Could you check a few things on this model? Use its own coordinates, in mm. A direction names the side the tool comes from. Give positions to 0.01 mm unless a question says otherwise; leave off trailing zeros. Order: outer loops, then holes, each group sorted by start corner. A loop starts at its lowest first (then second) coordinate and runs counter-clockwise, first axis right, second up. Notation, with made-up numbers: M 69.5,52 L 88.5,52 A12 cw 88.5,59 Z; hole C -33.75,40 d4. An arc over 180 degrees is marked long. Use a Markdown table: item, result. Add a question column.
Item 1: For faces 4 (the face through (35.821, 4.493, -11.113)), 5 (the face through (43.361, 2, -2)), 6 (the face through (33, 2, -12)), which set-ups out of +Z, -Z, +X, -X, +Y, -Y let a thin tool reach every point of the face, with its end or its side?
Item 2: If I drill on L1, parallel to Z at x = -24.5, y = 2.8; L2, parallel to Z at x = 34, y = 3; L3, parallel to X at y = 0.85, z = 5.5, over which ranges is the centre line in solid material (lowest first)? Write a range as from..to.
Item 3: Suppose I cut it at C-C on y = 1.15. Count the separate pieces of the cut face and the enclosed holes in it, plus the area to 3 significant figures.
Item 4: If we mould it in two halves opening along Z, with no side actions, what happens to faces 1 (the face through (34, 2, 7)), 2 (the face through (42, 2.5, 15)), 3 (the face through (-21.549, 3.455, -13.824))? For each: released by +Z, released by -Z, zero draft, split by the parting line, or undercut.
Item 5: Suppose I cut it at A-A on x = 15.5. Write out the boundary of the cut face in (y, z), plus the area to 3 significant figures.
Item 6: I'm going to push flat-ended pins straight in: pin 1 Ø1 at (x, y) = (34, 3.5) entering from +Z; pin 2 Ø0.8 at (y, z) = (1.5, -14) entering from +X; pin 3 Ø1 at (x, y) = (0.5, 4) entering from -Z. Where does each tip first touch, or does it pass through?
Item 7: Suppose I cut it at B-B on z = -0.5. Write out the boundary of the cut face in (x, y).
from build123d import *

# Parameters (mm, degrees)
SKETCH1_W                = 84.6
SKETCH1_H                = 27
BOSS_EXTRUDE1_DEPTH      = 5
CUT_EXTRUDE1_REACH       = 50.274
BOSS_EXTRUDE3_START      = 2
BOSS_EXTRUDE3_DEPTH      = 2
CUT_EXTRUDE3_START       = -2.5
CUT_EXTRUDE3_DEPTH       = 2.5
CUT_EXTRUDE5_START       = -2.5
CUT_EXTRUDE5_DEPTH       = 46.773999335
BOSS_EXTRUDE4_DEPTH      = 2.5
BOSS_EXTRUDE5_START      = -2.5
BOSS_EXTRUDE5_DEPTH      = 2.5
CUT_EXTRUDE2_OUTLINE_R   = 0.5
CUT_EXTRUDE2_OUTLINE_R_2 = 0.499999992
CUT_EXTRUDE2_DEPTH       = 5
SKETCH15_R               = 0.5
CUT_EXTRUDE6_DEPTH       = 50.255349811
SKETCH16_R               = 0.45
BOSS_EXTRUDE6_DEPTH      = 1


# Read off the part's stored shape, not the designer's step: Cut-Extrude2
with BuildPart() as part:
    # Sketch1 → Boss-Extrude1 (new body)
    with BuildSketch(Plane(origin=(0, 0, 0), x_dir=(1, 0, 0), z_dir=(0, 1, 0))):
        with Locations((3.06331835, 2.23366963)):
            Rectangle(SKETCH1_W, SKETCH1_H)
    extrude(amount=BOSS_EXTRUDE1_DEPTH)

    # Sketch3 → Cut-Extrude1 (cut, up to next)
    with BuildSketch(Plane(origin=(0, 0, 0), x_dir=(1, 0, 0), z_dir=(0, 1, 0)), mode=Mode.PRIVATE) as cut_extrude1_sk1:
        with BuildLine():
            Line((32.919678843, -9.163538235), (-27.280321157, -9.163538235))
            Line((-27.280321157, -9.163538235), (-27.280321157, -7.45100236))
            ThreePointArc((-27.280321157, -7.45100236), (-27.780321157, -6.95100236), (-28.280321157, -7.45100236))
            Line((-28.280321157, -7.45100236), (-28.280321157, -9.262483826))
            Line((-28.280321157, -9.262483826), (-34.233122665, -9.262483826))
            Line((-34.233122665, -9.262483826), (-34.233122665, -4.266133774))
            ThreePointArc((-34.233122665, -4.266133774), (-34.380628165, -3.910023997), (-34.736737941, -3.762518498))
            Line((-34.736737941, -3.762518498), (-37.233015401, -3.762518498))
            Line((-37.233015401, -3.762518498), (-37.233015401, 8.229171698))
            Line((-37.233015401, 8.229171698), (-34.736926038, 8.23003019))
            ThreePointArc((-34.736926038, 8.23003019), (-34.380928238, 8.377596904), (-34.233483972, 8.733645436))
            Line((-34.233483972, 8.733645436), (-34.233483972, 13.729919004))
            Line((-34.233483972, 13.729919004), (-31.31194803, 13.729919004))
            Line((-31.31194803, 13.729919004), (-31.31194803, 12.633776758))
            ThreePointArc((-31.31194803, 12.633776758), (-29.91194803, 11.233776758), (-28.51194803, 12.633776758))
            Line((-28.51194803, 12.633776758), (-28.51194803, 13.730371923))
            Line((-28.51194803, 13.730371923), (-21.508882253, 13.730371923))
            Line((-21.508882253, 13.730371923), (-20.139800412, 10.535595096))
            ThreePointArc((-20.139800412, 10.535595096), (-19.954180397, 10.31357804), (-19.676997597, 10.230415195))
            Line((-19.676997597, 10.230415195), (25.793967371, 10.230415195))
            ThreePointArc((25.793967371, 10.230415195), (26.055680662, 10.259428791), (26.266864173, 10.416709306))
            Line((26.266864173, 10.416709306), (27.639394616, 13.61080525))
            Line((27.639394616, 13.61080525), (34.4513038, 13.61080525))
            Line((34.4513038, 13.61080525), (34.4513038, 12.512891353))
            ThreePointArc((34.4513038, 12.512891353), (35.8513038, 11.112891353), (37.2513038, 12.512891353))
            Line((37.2513038, 12.512891353), (37.2513038, 13.612023992))
            Line((37.2513038, 13.612023992), (40.361611802, 13.612023992))
            Line((40.361611802, 13.612023992), (40.361611802, 8.61576965))
            ThreePointArc((40.361611802, 8.61576965), (40.509053891, 8.259723294), (40.865047712, 8.112154406))
            Line((40.865047712, 8.112154406), (43.361137065, 8.111265408))
            Line((43.361137065, 8.111265408), (43.361137065, -3.763055079))
            Line((43.361137065, -3.763055079), (40.86393165, -3.763055079))
            ThreePointArc((40.86393165, -3.763055079), (40.507821873, -3.910560578), (40.360316374, -4.266670355))
            Line((40.360316374, -4.266670355), (40.360316374, -9.163538235))
            Line((40.360316374, -9.163538235), (34.019678843, -9.163538235))
            Line((34.019678843, -9.163538235), (34.019678843, -7.715606668))
            ThreePointArc((34.019678843, -7.715606668), (33.469678843, -7.165606668), (32.919678843, -7.715606668))
            Line((32.919678843, -7.715606668), (32.919678843, -9.163538235))
        make_face()
    cut_extrude1_tool1 = extrude(cut_extrude1_sk1.sketch, amount=CUT_EXTRUDE1_REACH, mode=Mode.PRIVATE) & part.part
    add(cut_extrude1_tool1.solids().sort_by_distance((3.012517, 0, -1.196465))[0], mode=Mode.SUBTRACT)

    # Sketch3<5> → Boss-Extrude3 (add)
    with BuildSketch(Plane(origin=(0, 0, 0), x_dir=(1, 0, 0), z_dir=(0, 1, 0)).offset(BOSS_EXTRUDE3_START)):
        with BuildLine():
            Line((26.852330657, -9.163538235), (32.919678843, -9.163538235))
            Line((32.919678843, -9.163538235), (32.919678843, -7.715606668))
            ThreePointArc((32.919678843, -7.715606668), (33.469678843, -7.165606668), (34.019678843, -7.715606668))
            Line((34.019678843, -7.715606668), (34.019678843, -9.163538235))
            Line((34.019678843, -9.163538235), (40.360316374, -9.163538235))
            Line((40.360316374, -9.163538235), (40.360316374, -4.950942773))
            Line((40.360316374, -4.950942773), (27.852330657, -4.950942773))
            ThreePointArc((27.852330657, -4.950942773), (27.145223876, -5.243835992), (26.852330657, -5.950942773))
            Line((26.852330657, -5.950942773), (26.852330657, -9.163538235))
        make_face()
        with BuildLine():
            Line((-27.280321157, -9.163538235), (-22.401406955, -9.163538235))
            Line((-22.401406955, -9.163538235), (-22.401406955, -5.777559213))
            ThreePointArc((-22.401406955, -5.777559213), (-22.692236098, -5.07252255), (-23.395560348, -4.777576304))
            Line((-23.395560348, -4.777576304), (-34.233122665, -4.777576304))
            Line((-34.233122665, -4.777576304), (-34.233122665, -9.262483826))
            Line((-34.233122665, -9.262483826), (-28.280321157, -9.262483826))
            Line((-28.280321157, -9.262483826), (-28.280321157, -7.45100236))
            ThreePointArc((-28.280321157, -7.45100236), (-27.780321157, -6.95100236), (-27.280321157, -7.45100236))
            Line((-27.280321157, -7.45100236), (-27.280321157, -9.163538235))
        make_face()
        with BuildLine():
            Line((26.400356299, 10.727366647), (40.361611802, 10.727366647))
            Line((40.361611802, 10.727366647), (40.361611802, 13.612023992))
            Line((40.361611802, 13.612023992), (37.2513038, 13.612023992))
            Line((37.2513038, 13.612023992), (37.2513038, 12.512891353))
            ThreePointArc((37.2513038, 12.512891353), (35.8513038, 11.112891353), (34.4513038, 12.512891353))
            Line((34.4513038, 12.512891353), (34.4513038, 13.61080525))
            Line((34.4513038, 13.61080525), (27.639394616, 13.61080525))
            Line((27.639394616, 13.61080525), (26.400356299, 10.727366647))
        make_face()
        with BuildLine():
            Line((-34.233483972, 13.729919004), (-34.233483972, 10.733923481))
            Line((-34.233483972, 10.733923481), (-20.224791573, 10.733923481))
            Line((-20.224791573, 10.733923481), (-21.508882253, 13.730371923))
            Line((-21.508882253, 13.730371923), (-28.51194803, 13.730371923))
            Line((-28.51194803, 13.730371923), (-28.51194803, 12.633776758))
            ThreePointArc((-28.51194803, 12.633776758), (-29.91194803, 11.233776758), (-31.31194803, 12.633776758))
            Line((-31.31194803, 12.633776758), (-31.31194803, 13.729919004))
            Line((-31.31194803, 13.729919004), (-34.233483972, 13.729919004))
        make_face()
    extrude(amount=BOSS_EXTRUDE3_DEPTH)

    # Sketch13 → Cut-Extrude3 (cut)
    with BuildSketch(Plane(origin=(0, 5, 0), x_dir=(1, 0, 0), z_dir=(0, 1, 0)).offset(CUT_EXTRUDE3_START)):
        with BuildLine():
            Line((-22.367370549, 15.73366963), (-20.139800412, 10.535595096))
            ThreePointArc((-20.139800412, 10.535595096), (-19.954180397, 10.31357804), (-19.676997597, 10.230415195))
            Line((-19.676997597, 10.230415195), (25.793967371, 10.230415195))
            ThreePointArc((25.793967371, 10.230415195), (26.055680662, 10.259428791), (26.266864173, 10.416709306))
            Line((26.266864173, 10.416709306), (28.551607662, 15.73366963))
            Line((28.551607662, 15.73366963), (-22.367370549, 15.73366963))
        make_face()
    extrude(amount=CUT_EXTRUDE3_DEPTH, mode=Mode.SUBTRACT)

    # Sketch13<4> → Cut-Extrude5 (cut, through all)
    with BuildSketch(Plane(origin=(0, 5, 0), x_dir=(1, 0, 0), z_dir=(0, 1, 0)).offset(CUT_EXTRUDE5_START)):
        with BuildLine():
            Line((-34.233483972, 8.733645436), (-34.233483972, 15.73366963))
            Line((-34.233483972, 15.73366963), (-39.23668165, 15.73366963))
            Line((-39.23668165, 15.73366963), (-39.23668165, 8.228482568))
            Line((-39.23668165, 8.228482568), (-34.736926038, 8.23003019))
            ThreePointArc((-34.736926038, 8.23003019), (-34.380928238, 8.377596904), (-34.233483972, 8.733645436))
        make_face()
        with BuildLine():
            Line((45.36331835, 8.110552318), (45.36331835, 15.73366963))
            Line((45.36331835, 15.73366963), (40.361611802, 15.73366963))
            Line((40.361611802, 15.73366963), (40.361611802, 8.61576965))
            ThreePointArc((40.361611802, 8.61576965), (40.509053891, 8.259723294), (40.865047712, 8.112154406))
            Line((40.865047712, 8.112154406), (45.36331835, 8.110552318))
        make_face()
    extrude(amount=-CUT_EXTRUDE5_DEPTH, mode=Mode.SUBTRACT)

    # Sketch13<7> → Boss-Extrude4 (add)
    with BuildSketch(Plane(origin=(0, 5, 0), x_dir=(1, 0, 0), z_dir=(0, 1, 0))):
        with BuildLine():
            Line((26.149886209, -16.077855955), (28.210353336, -11.26633037))
            Line((28.210353336, -11.26633037), (-22.112103374, -11.26633037))
            Line((-22.112103374, -11.26633037), (-20.033790882, -16.079245346))
            ThreePointArc((-20.033790882, -16.079245346), (-19.849433129, -16.298824073), (-19.574759994, -16.381026671))
            Line((-19.574759994, -16.381026671), (25.690257845, -16.381026671))
            ThreePointArc((25.690257845, -16.381026671), (25.965562547, -16.298408177), (26.149886209, -16.077855955))
        make_face()
    extrude(amount=-BOSS_EXTRUDE4_DEPTH)

    # Sketch13<8> → Boss-Extrude5 (add)
    with BuildSketch(Plane(origin=(0, 5, 0), x_dir=(1, 0, 0), z_dir=(0, 1, 0)).offset(BOSS_EXTRUDE5_START)):
        with BuildLine():
            Line((-34.498583653, -18.273630424), (-34.498583653, -11.26633037))
            Line((-34.498583653, -11.26633037), (-39.23668165, -11.26633037))
            Line((-39.23668165, -11.26633037), (-39.23668165, -18.526779589))
            Line((-39.23668165, -18.526779589), (-34.736829858, -18.526779589))
            ThreePointArc((-34.736829858, -18.526779589), (-34.567511978, -18.447444803), (-34.498583653, -18.273630424))
        make_face()
        with BuildLine():
            Line((45.36331835, -11.26633037), (40.594578125, -11.26633037))
            Line((40.594578125, -11.26633037), (40.594578125, -18.273630424))
            ThreePointArc((40.594578125, -18.273630424), (40.674379022, -18.458317374), (40.863562472, -18.526779589))
            Line((40.863562472, -18.526779589), (45.36331835, -18.526779589))
            Line((45.36331835, -18.526779589), (45.36331835, -11.26633037))
        make_face()
    extrude(amount=-BOSS_EXTRUDE5_DEPTH)

    # Cut-Extrude2 outline → Cut-Extrude2 (cut)
    with BuildSketch(Plane.XZ.offset(-5)):
        with Locations((30.98643714, -12.338409577)):
            Circle(CUT_EXTRUDE2_OUTLINE_R)
        with Locations((-25.04708137, -12.338409577)):
            Circle(CUT_EXTRUDE2_OUTLINE_R)
        with Locations((-24.430322115, 6.911590423)):
            Circle(CUT_EXTRUDE2_OUTLINE_R)
        with Locations((-36.73668165, -11.98366963)):
            Circle(CUT_EXTRUDE2_OUTLINE_R)
        with Locations((-15.856255457, -13.23366963)):
            Circle(CUT_EXTRUDE2_OUTLINE_R)
        with Locations((22.035256025, -13.23366963)):
            Circle(CUT_EXTRUDE2_OUTLINE_R_2)
        with Locations((42.86331835, -11.98366963)):
            Circle(CUT_EXTRUDE2_OUTLINE_R)
        with Locations((-36.73668165, 7.51633037)):
            Circle(CUT_EXTRUDE2_OUTLINE_R)
        with Locations((42.86331835, 7.51633037)):
            Circle(CUT_EXTRUDE2_OUTLINE_R)
    extrude(amount=CUT_EXTRUDE2_DEPTH, mode=Mode.SUBTRACT)

    # Sketch15 → Cut-Extrude6 (cut, through all)
    with BuildSketch(Plane(origin=(0, 5, 0), x_dir=(1, 0, 0), z_dir=(0, 1, 0))):
        with Locations(Location((-15.856255457, -14.031026671, 0), (0, 0, 270))):
            Circle(SKETCH15_R)
        with Locations(Location((22.039147194, -14.031026671, 0), (0, 0, 270))):
            Circle(SKETCH15_R)
        with Locations(Location((-36.73668165, -15.276779589, 0), (0, 0, 270))):
            Circle(SKETCH15_R)
        with Locations(Location((42.86331835, -15.276779589, 0), (0, 0, 270))):
            Circle(SKETCH15_R)
    extrude(amount=-CUT_EXTRUDE6_DEPTH, mode=Mode.SUBTRACT)

    # Sketch16 → Boss-Extrude6 (add)
    with BuildSketch(Plane(origin=(0, 4, 0), x_dir=(1, 0, 0), z_dir=(0, 1, 0))):
        with Locations(Location((38.269677885, 11.588409577, 0), (0, 0, 90))):
            Circle(SKETCH16_R)
        with Locations(Location((-32.330322115, -7.661590423, 0), (0, 0, 90))):
            Circle(SKETCH16_R)
    extrude(amount=BOSS_EXTRUDE6_DEPTH)


solid = part.part
Findings below:
| question | item | result |
|---|---|---|
| 1 | face 4 | +Y |
| 1 | face 5 | +Y, -Y |
| 1 | face 6 | -Y |
| 2 | L1 | z = -15.73..-10.73, 4.78..6.42, 7.41..11.27 |
| 2 | L2 | z = -15.73..-10.73, 4.95..11.27 |
| 2 | L3 | x = -39.24..-34.23, 40.36..45.36 |
| 3 | separate pieces | 2 |
| 3 | enclosed holes | 6 |
| 3 | area | 678 mm^2 |
| 4 | face 1 | undercut |
| 4 | face 2 | zero draft |
| 4 | face 3 | released by -Z |
| 5 | outline | M 0,-15.73 L 2.5,-15.73 L 2.5,-10.23 L 0,-10.23 Z; M 0,9.16 L 5,9.16 L 5,16.38 L 2.5,16.38 L 2.5,11.27 L 0,11.27 Z |
| 5 | area | 37.1 mm^2 |
| 6 | pin 1 | stops at z = 11.27 |
| 6 | pin 2 | stops at x = 40.36 |
| 6 | pin 3 | stops at z = 9.16 |
| 7 | outline | M -39.24,0 L -37.23,0 L -37.23,5 L -39.24,5 Z; M 43.36,0 L 45.36,0 L 45.36,5 L 43.36,5 Z |
